Work out the finished part from the listing and answer in its coordinate system (mm). Coordinates: 2 decimals unless noted, no trailing zeros. Loops run counter-clockwise (first coordinate to the right, second up) from the corner with the lowest first, then second, coordinate; pieces in that order, holes last. Notation, with made-up numbers: M 87.5,-27.75 L 97.5,-27.75 A25 ccw 97.5,5.25 Z; hole C 18,-30 d7. An arc over 180 degrees is marked long. Write each question's results on one line, items separated by ' | '.
Autodesk Inventor part; units mm, degrees
ref_plane "YZ Plane" through (0, 0, 0) normal (1, 0, 0) x (0, 1, 0)
ref_plane "XZ Plane" through (0, 0, 0) normal (0, 1, 0) x (-1, 0, 0)
ref_plane "XY Plane" through (0, 0, 0) normal (0, 0, 1) x (1, 0, 0)
sketch "Sketch1" plane through (0, 0, 0) normal (0, 1, 0) x (-1, 0, 0)
  line L0 (39.6875, -38.1) -> (-39.6875, -38.1)
  line L1 (-39.6875, -38.1) -> (-39.6875, 38.1)
  line L2 (-39.6875, 38.1) -> (39.6875, 38.1)
  line L3 (39.6875, 38.1) -> (39.6875, -38.1)
  line L4 (39.6875, -38.1) -> (-39.6875, 38.1) construction
  line L5 (-39.6875, -38.1) -> (39.6875, 38.1) construction
  point P0 (0, 0)
  dimension "d0" = 76.2
  dimension "d1" = 79.375
extrude "Extrusion1" add sketch "Sketch1" along normal mid plane 6.35
sketch "Sketch2" plane through (0, 3.175, 0) normal (0, 1, 0) x (1, 0, 0)
  line L0 (-39.6875, 38.1) -> (-39.6875, -38.1)
  line L1 (39.6875, -38.1) -> (39.6875, 38.1)
  line L2 (39.6875, 38.1) -> (-39.6875, 38.1)
  line L3 (-39.6875, -38.1) -> (39.6875, -38.1)
  point P0 (0, 0)
  point P1 (-30.1625, 25.4)
  point P2 (-30.1625, -25.4)
  point P3 (30.1625, 25.4)
  point P4 (30.1625, -25.4)
  dimension "d4" = 9.525
  dimension "d5" = 9.525
  dimension "d6" = 9.525
  dimension "d7" = 9.525
  dimension "d8" = 12.7
  dimension "d9" = 12.7
  dimension "d10" = 12.7
  dimension "d11" = 12.7
hole "Hole1" at (-30.1625, 3.175, -25.4) at (-30.1625, 3.175, 25.4) at (30.1625, 3.175, -25.4) at (30.1625, 3.175, 25.4) direction (0, -1, 0) diameter 5.3086 end through all
sketch "Sketch3" plane through (0, 3.175, 0) normal (0, 1, 0) x (1, 0, 0)
  circle A0 centre (30.1625, 25.4) radius 2.6543
  circle A1 centre (-30.1625, 25.4) radius 2.6543
  circle A2 centre (-30.1625, -25.4) radius 2.6543
  circle A3 centre (30.1625, -25.4) radius 2.6543
  line L0 (39.6875, -38.1) -> (39.6875, 38.1)
  line L1 (39.6875, 38.1) -> (-39.6875, 38.1)
  line L2 (-39.6875, 38.1) -> (-39.6875, -38.1)
  line L3 (-39.6875, -38.1) -> (39.6875, -38.1)
  line L4 (-30.1625, 25.4) -> (-26.9875, 25.4) construction
  line L5 (-30.1625, 22.7457) -> (-26.9875, 22.7457)
  line L6 (-26.9875, 28.0543) -> (-30.1625, 28.0543)
  arc A4 (-30.1625, 28.0543) -> (-30.1625, 22.7457) centre (-30.1625, 25.4) ccw
  arc A5 (-26.9875, 22.7457) -> (-26.9875, 28.0543) centre (-26.9875, 25.4) ccw
  line L7 (-30.1625, -25.4) -> (-26.9875, -25.4) construction
  line L8 (-30.1625, -22.7457) -> (-26.9875, -22.7457)
  line L9 (-26.9875, -28.0543) -> (-30.1625, -28.0543)
  arc A6 (-30.1625, -22.7457) -> (-30.1625, -28.0543) centre (-30.1625, -25.4) ccw
  arc A7 (-26.9875, -28.0543) -> (-26.9875, -22.7457) centre (-26.9875, -25.4) ccw
  point P0 (0, 0)
  point P1 (-28.575, 25.4)
  point P2 (-28.575, -25.4)
  dimension "d19" = 3.175
  dimension "d20" = 3.175
extrude "Extrusion2" cut sketch "Sketch3" against normal blind 6.35 contours A1 L6 A5 L5 | A2 L8 A7 L9
sketch "Sketch4" plane through (0, 3.175, 0) normal (0, 1, 0) x (1, 0, 0)
  line L0 (39.6875, -38.1) -> (39.6875, 38.1)
  line L1 (39.6875, 38.1) -> (-39.6875, 38.1)
  line L2 (-39.6875, -38.1) -> (39.6875, -38.1)
  circle A0 centre (30.1625, 25.4) radius 2.6543
  circle A1 centre (30.1625, -25.4) radius 2.6543
  point P0 (0, 0)
  point P1 (27.6625, 10)
  point P2 (27.6625, -10)
  dimension "d33" = 15.4
  dimension "d34" = 2.5
  dimension "d35" = 15.4
hole "Hole2" at (27.6625, 3.175, -10) at (27.6625, 3.175, 10) direction (0, -1, 0) diameter 5.5 end through all
equation "\"d20\" = d19"
properties part number "X-Axis_End_Plate_LM3004" material "Polycarbonate, Smoke"
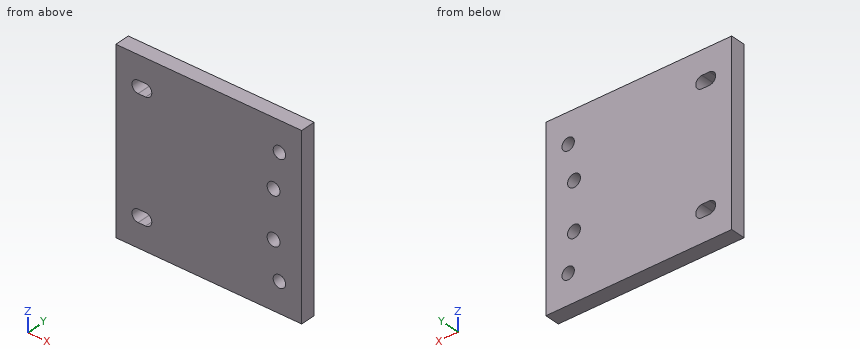
1) Straight lines are drawn through the part: probe 1 along X at (y, z) = (0.75, -25.4); probe 2 along Z at (x, y) = (-28.5, 2.5); probe 3 along X at (y, z) = (1, -10). For each, find the intervals that lie inside material, in ascending order. Write a range as [from, to].
Check result:
probe 1: [-39.69, -32.82], [-24.33, 27.51], [32.82, 39.69] | probe 2: [-38.1, -28.05], [-22.75, 22.75], [28.05, 38.1] | probe 3: [-39.69, 24.91], [30.41, 39.69]
2) Find section B-B, the plane z = -25.4. Give the vertices of the cut face in (x, y) (1 decimal), and give its area (3 significant figures).
Check result:
outline: M -39.7,-3.2 L -32.8,-3.2 L -32.8,3.2 L -39.7,3.2 Z; M -24.3,-3.2 L 27.5,-3.2 L 27.5,3.2 L -24.3,3.2 Z; M 32.8,-3.2 L 39.7,-3.2 L 39.7,3.2 L 32.8,3.2 Z | area: 416 mm^2
3) Given pin 1 Ø7 at (x, z) = (27.66, -10) entering from -Y (3 decimals); pin 2 Ø5 at (x, z) = (27.66, 10) entering from -Y, each flat-ended and moving along its own axis, determine where each tip first touches the part or whether it passes through.
Check result:
pin 1: y = -3.175 | pin 2: through
4) Find section A-A, the plane x = -28. Give the vertices of the cut face in (y, z) (3 decimals).
Check result:
outline: M -3.175,-38.1 L 3.175,-38.1 L 3.175,-28.054 L -3.175,-28.054 Z; M -3.175,-22.746 L 3.175,-22.746 L 3.175,22.746 L -3.175,22.746 Z; M -3.175,28.054 L 3.175,28.054 L 3.175,38.1 L -3.175,38.1 Z
5) Find section C-C, the plane z = -10. Give the vertices of the cut face in (x, y) (1 decimal).
Check result:
outline: M -39.7,-3.2 L 24.9,-3.2 L 24.9,3.2 L -39.7,3.2 Z; M 30.4,-3.2 L 39.7,-3.2 L 39.7,3.2 L 30.4,3.2 Z
6) Find section D-D, the plane y = 0.25. Give the vertices of the cut face in (x, z), and give its area (3 significant figures).
Check result:
outline: M -39.69,-38.1 L 39.69,-38.1 L 39.69,38.1 L -39.69,38.1 Z; hole M -30.16,-28.05 L -26.99,-28.05 A2.65 ccw -26.99,-22.75 L -30.16,-22.75 A2.65 ccw Z; hole M -30.16,22.75 L -26.99,22.75 A2.65 ccw -26.99,28.05 L -30.16,28.05 A2.65 ccw Z; hole C 27.66,-10 d5.5; hole C 27.66,10 d5.5; hole C 30.16,-25.4 d5.31; hole C 30.16,25.4 d5.31 | area: 5,880 mm^2
